```python
from build123d import *

# Parameters (mm, degrees)
SKETCH_1_R          = 2
EXTRUDE_1_DEPTH     = 16
SKETCH_2_R          = 3.3
EXTRUDE_2_DEPTH     = 2.7
FILLET_1_R          = 1
CHAMFER_1_SIZE      = 0.5
SKETCH_3_W          = 4
SKETCH_3_H          = 1
SKETCH_3_W_2        = 1
SKETCH_3_H_2        = 4
CUT_EXTRUDE_1_DEPTH = 1
CHAMFER_2_SIZE      = 1


with BuildPart() as part:
    # 草图1 → 凸台-拉伸1 (new body)
    with BuildSketch(Plane(origin=(0, 0, 0), x_dir=(1, 0, 0), z_dir=(0, 1, 0))):
        with Locations(Location((0, 0, 0), (0, 0, 270))):
            Circle(SKETCH_1_R)
    extrude(amount=EXTRUDE_1_DEPTH)

    # 草图2 → 凸台-拉伸2 (add)
    with BuildSketch(Plane(origin=(0, 16, 0), x_dir=(1, 0, 0), z_dir=(0, 1, 0))):
        with Locations(Location((0, 0, 0), (0, 0, 90))):
            Circle(SKETCH_2_R)
    extrude(amount=EXTRUDE_2_DEPTH)

    # 圆角1
    fillet_1_edges = [part.edges().sort_by_distance(p)[0] for p in [
        (0, 18.7, 3.3),
    ]]
    fillet(fillet_1_edges, radius=FILLET_1_R)

    # 倒角1
    chamfer_1_edges = [part.edges().sort_by_distance(p)[0] for p in [
        (0, 0, -2),
    ]]
    chamfer(chamfer_1_edges, length=CHAMFER_1_SIZE)

    # 草图3 → 切除-拉伸-薄壁1 (cut)
    with BuildSketch(Plane(origin=(0, 18.7, 0), x_dir=(1, 0, 0), z_dir=(0, 1, 0))):
        Rectangle(SKETCH_3_W, SKETCH_3_H)
        Rectangle(SKETCH_3_W_2, SKETCH_3_H_2)
    extrude(amount=-CUT_EXTRUDE_1_DEPTH, mode=Mode.SUBTRACT)

    # 倒角2
    chamfer_2_edges = [part.edges().sort_by_distance(p)[0] for p in [
        (0, 17.7, 2),
        (2, 17.7, 0),
        (0, 17.7, -2),
        (-2, 17.7, 0),
    ]]
    chamfer(chamfer_2_edges, length=CHAMFER_2_SIZE - 0.0001)  # a hair under: the kernel refuses the full size


solid = part.part
```
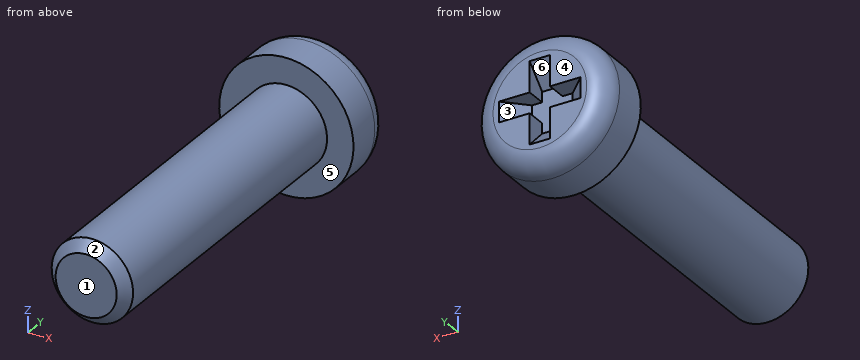
The listing builds one solid part. Answer for the finished solid, in the listing's coordinates (mm). Face numbers are marked on the shaded views. A direction names the side the tool comes from. Give positions to 0.01 mm unless a question says otherwise; leave off trailing zeros. Order: outer loops, then holes, each group sorted by start corner. A loop starts at its lowest first (then second) coordinate and runs counter-clockwise, first axis right, second up.
Item 1: Which of the six approach directions +Z, -Z, +X, -X, +Y, -Y give full straight-line access (tool end or side, diameter ignored) to the marked faces 4, 5 and 6?
From the geometry:
face 4: +Z, -Z, +X, -X, +Y
face 5: -Y
face 6: +Y
Item 2: The part is cut by section C-C, the plane y = 14.25. Give the vertices of the cut face in (x, z).
From the geometry:
outline: circle Ø4 at (0, 0)
Item 3: For a pull along X with two mould halves and no side action, classify the marked faces 1, 2 and 3 as pulls with the +X half, pulls with the -X half, needs draft (parallel to the pull), parting line crosses it, or undercut.
From the geometry:
face 1: needs draft
face 2: parting line crosses it
face 3: undercut
Item 4: Find the intervals of material crossed by probe 1 along Y at (x, z) = (-2.25, -0.25); probe 2 along X at (y, z) = (16.5, 2); probe 3 along X at (y, z) = (17, 2.5), in increasing order.
From the geometry:
probe 1: y = 16 to 18.7
probe 2: x = -2.62 to 2.62
probe 3: x = -2.15 to 2.15
Item 5: Given pin 1 Ø3 at (x, z) = (1, 2.5) entering from -Y; pin 2 Ø0.5 at (y, z) = (18, 1) entering from +X; pin 3 Ø0.8 at (x, y) = (1.5, 18.5) entering from -Z; pin 4 Ø2 at (y, z) = (6.5, 0) entering from +X, each flat-ended and moving along its own axis, determine where each tip first touches the part or whether it passes through.
From the geometry:
pin 1: stops at y = 0
pin 2: stops at x = 3.19
pin 3: stops at z = -2.92
pin 4: stops at x = 2
